from build123d import *

# Parameters (mm, degrees)
F0_W     = 203
F0_H     = 108
F1_DEPTH = 5
F2_R     = 40
F3_DEPTH = 180
F4_R     = 35
F5_DEPTH = 180
F6_R     = 10
F7_R     = 2


with BuildPart() as f1:
    # F0 (on Top) → F1 (new body)
    with BuildSketch(Plane.XY):
        Rectangle(F0_W, F0_H)
    extrude(amount=F1_DEPTH)

    # F2 (on face) → F3 (join)
    with BuildSketch(Plane.XY.offset(5)):
        Circle(F2_R)
    extrude(amount=F3_DEPTH)

    # F4 (on face) → F5 (cut)
    with BuildSketch(Plane.XY.offset(185)):
        Circle(F4_R)
    extrude(amount=-F5_DEPTH, mode=Mode.SUBTRACT)

    # F6
    f6_edges = [f1.edges().sort_by_distance(p)[0] for p in [
        (101.5, -54, 2.5),
        (101.5, 54, 2.5),
        (-101.5, 54, 2.5),
        (-101.5, -54, 2.5),
    ]]
    fillet(f6_edges, radius=F6_R)

    # F7
    f7_edges = [f1.edges().sort_by_distance(p)[0] for p in [
        (-40, 0, 185),
    ]]
    fillet(f7_edges, radius=F7_R)


solid = f1.part
Design review of the part built by this model. Coordinates are the model's own, in mm. A direction names the side the tool comes from. Round coordinates to 2 decimals unless told otherwise and drop trailing zeros. Loops run counter-clockwise (first coordinate to the right, second up) from the corner with the lowest first, then second, coordinate; pieces in that order, holes last. Notation, with made-up numbers: M 20,-34.75 L 39,-34.75 A37 cw 39,3.25 Z; hole C 85.25,-30.5 d7. An arc over 180 degrees is marked long. Answer as a JSON object with one key per item and string values.
Item 1: The part is to be moulded in two halves that separate along X. For faces 1 (the cylindrical face through (-28, -21, 96)), 2 (the flat face through (-1, -54, 2)), 3 (the cylindrical face through (-98.65, 50.99, 2.54)), 4 (the flat face through (0, 0, 5)), say which applies: pulls with the +X half, pulls with the -X half, needs draft (parallel to the pull), parting line crosses it, or undercut.
Answer sheet:
{"face 1": "undercut", "face 2": "needs draft", "face 3": "pulls with the -X half", "face 4": "undercut"}
Item 2: Wall thickness on L1, parallel to Y at x = 0, z = 69.5; L2, parallel to X at y = 3, z = 164.5: over which ranges is each line inside the solid? List them lowest first. Write a range as from..to.
Answer sheet:
{"L1": "y = -40..-35, 35..40", "L2": "x = -39.89..-34.87, 34.87..39.89"}
Item 3: We need section B-B on x = 0. Give the boundary of the cut face in (y, z).
Answer sheet:
{"outline": "M -54,0 L 54,0 L 54,5 L 40,5 L 40,183 A2 ccw 38,185 L 35,185 L 35,5 L -35,5 L -35,185 L -38,185 A2 ccw -40,183 L -40,5 L -54,5 Z"}
Item 4: We need section D-D on x = 66. Give the boundary of the cut face in (y, z).
Answer sheet:
{"outline": "M -54,0 L 54,0 L 54,5 L -54,5 Z"}
Item 5: We need section A-A on y = 0. Give the boundary of the cut face in (x, z), and give its area (3 significant figures).
Answer sheet:
{"outline": "M -101.5,0 L 101.5,0 L 101.5,5 L 40,5 L 40,183 A2 ccw 38,185 L 35,185 L 35,5 L -35,5 L -35,185 L -38,185 A2 ccw -40,183 L -40,5 L -101.5,5 Z", "area": "2,810 mm^2"}
Item 6: Machinability: for faces 5 (the cylindrical face through (98.49, -51.15, 2.54)), 6 (the cylindrical face through (-8.67, -39.05, 92.75)), which of the approach directions +Z, -Z, +X, -X, +Y, -Y give a long, thin tool a straight path to every point of the face, cutting with its end or side? Answer none if there is none.
Answer sheet:
{"face 5": "+Z, -Z, +X, -Y", "face 6": "+Z"}
Item 7: Clearance check with flat-ended pins moving along their axes: P1, Ø12, axis at x = 63.5, y = -40.5, coming from the -Z side; P2, Ø2, axis at x = 62.5, y = 6, coming from the +Z side; P3, Ø4, axis at y = -5, z = 40.5, coming from the +X side; P4, Ø10, axis at y = 36, z = 133, coming from the +X side. State where each tip first meets the part, or that it passes through.
Answer sheet:
{"P1": "stops at z = 0", "P2": "stops at z = 5", "P3": "stops at x = 39.89", "P4": "stops at x = 25.28"}
Item 8: We need section C-C on z = 29. Give the boundary of the cut face in (x, y), and give its area (3 significant figures).
Answer sheet:
{"outline": "C 0,0 d80; hole C 0,0 d70", "area": "1,180 mm^2"}
